Source: CAD feature listing. Evaluate the final solid. Frame: model axes, mm. Face numbers are marked on the shaded views. A direction names the side the tool comes from. Round coordinates to 2 decimals unless told otherwise and drop trailing zeros. Write each loop counter-clockwise with the first axis right and the second up, starting at its lowest first coordinate (ties: lowest second). Pieces come first, ordered by that corner, then holes. Notation, with made-up numbers: (81, -21) -> (89, -21) arc R32 ccw to (89, 9) -> close; hole circle Ø8 at (25.5, 44). An arc over 180 degrees is marked (long way). Put each result on its own line as item: value.
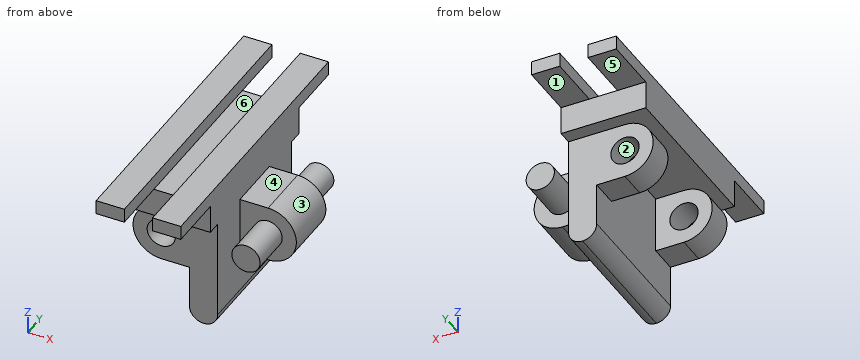
```python
from build123d import *

# Parameters (mm, degrees)
F0_W      = 5
F0_H      = 10
F0_R      = 2.5
F1_DEPTH  = 12.5
F2_DEPTH  = 5
F3_DEPTH  = 12.5
F4_DEPTH  = 7.5
F7_DEPTH  = 10
F8_R      = 2.5
F9_R      = 2.49999
F10_W     = 15
F10_H     = 30
F11_DEPTH = 5
F12_W     = 5
F12_H     = 50
F13_DEPTH = 2.5


# Not quite as in the source:
# - a fillet or chamfer is up to 0.001 mm smaller than in the source, because OpenCascade refuses the exact size


with BuildPart() as f1:
    # F0 (on Front) → F1 (new body)
    with BuildSketch(Plane.XZ):
        with Locations((7.5, 0)):
            Rectangle(F0_W, F0_H)
        with BuildLine():
            Line((5, 5), (0, 5))
            ThreePointArc((0, 5), (-5, 0), (0, -5))
            Line((0, -5), (5, -5))
            Line((5, -5), (5, 5))
        make_face()
        Circle(F0_R, mode=Mode.SUBTRACT)
    extrude(amount=F1_DEPTH)

    # F0 (on Front) → F2 (join)
    with BuildSketch(Plane.XZ):
        with BuildLine():
            Line((15, 5), (10, 5))
            Line((10, 5), (10, -5))
            Line((10, -5), (15, -5))
            ThreePointArc((15, -5), (20, 0), (15, 5))
        make_face()
        with Locations((15, 0)):
            Circle(F0_R, mode=Mode.SUBTRACT)
    extrude(amount=F2_DEPTH)

    # F0 (on Front) → F3 (join)
    with BuildSketch(Plane.XZ):
        with Locations((15, 0)):
            Circle(F0_R)
    extrude(amount=F3_DEPTH)

    # F0 (on Front) → F4 (cut)
    with BuildSketch(Plane.XZ):
        with BuildLine():
            Line((5, 5), (0, 5))
            ThreePointArc((0, 5), (-5, 0), (0, -5))
            Line((0, -5), (5, -5))
            Line((5, -5), (5, 5))
        make_face()
        Circle(F0_R, mode=Mode.SUBTRACT)
    extrude(amount=F4_DEPTH, mode=Mode.SUBTRACT)

    # F5: F1 across plane


with BuildPart() as f1_1:
    add(f1.part)
    add(f1.part.mirror(Plane.XZ))

    # F6 (on face) → F7 (join)
    with BuildSketch(Plane(origin=(0, 0, -5), x_dir=(1, 0, 0), z_dir=(0, 0, -1))):
        Polygon((10, 5), (10, 12.5), (5, 12.5), (5, 7.5), (5, -7.5), (5, -12.5), (10, -12.5), (10, -5), align=None)
    extrude(amount=F7_DEPTH)

    # F8
    f8_edges = [f1_1.edges().sort_by_distance(p)[0] for p in [
        (10, 0, -15),
    ]]
    fillet(f8_edges, radius=F8_R)

    # F9 (radius 2.5 in the source; OpenCascade refuses exactly that, so slightly less here)
    f9_edges = [f1_1.edges().sort_by_distance(p)[0] for p in [
        (5, 0, -15),
    ]]
    fillet(f9_edges, radius=F9_R)

    # F10 (on face) → F11 (join)
    with BuildSketch(Plane.XY.offset(5)):
        with Locations((2.5, 0)):
            Rectangle(F10_W, F10_H)
    extrude(amount=F11_DEPTH)

    # F12 (on face) → F13 (join)
    with BuildSketch(Plane.XY.offset(10)):
        with Locations((-2.5, 0)):
            Rectangle(F12_W, F12_H)
        with Locations((7.5, 0)):
            Rectangle(F12_W, F12_H)
    extrude(amount=F13_DEPTH)


solid = f1_1.part
```
Q1. Cut plane A-A on z = 0. Output: boundary loops of the cut face in (x, y), and give its area (3 significant figures).
Ans:
outline: (-5, -12.5) -> (-2.5, -12.5) -> (-2.5, -7.5) -> (-5, -7.5) -> close; (-5, 7.5) -> (-2.5, 7.5) -> (-2.5, 12.5) -> (-5, 12.5) -> close; (2.5, -12.5) -> (10, -12.5) -> (10, -5) -> (12.5, -5) -> (12.5, -12.5) -> (17.5, -12.5) -> (17.5, -5) -> (20, -5) -> (20, 5) -> (17.5, 5) -> (17.5, 12.5) -> (12.5, 12.5) -> (12.5, 5) -> (10, 5) -> (10, 12.5) -> (2.5, 12.5) -> (2.5, 7.5) -> (5, 7.5) -> (5, -7.5) -> (2.5, -7.5) -> close
area: 350 mm^2
Q2. Cut plane B-B on y = 19. Output: boundary loops of the cut face in (x, z).
Ans:
outline: (-5, 10) -> (0, 10) -> (0, 12.5) -> (-5, 12.5) -> close; (5, 10) -> (10, 10) -> (10, 12.5) -> (5, 12.5) -> close
Q3. Material intervals for line 1 (X direction, y = -10, z = 11.25); line 2 (Z direction, x = 4.75, y = -13); line 3 (Y direction, x = -3.5, z = 3.25), sorted ascending. Write a range as [from, to].
Ans:
line 1: x = [-5, 0], [5, 10]
line 2: z = [5, 10]
line 3: y = [-12.5, -7.5], [7.5, 12.5]
Q4. Reachability of the marked faces 4, 5 and 6 from +Z, -Z, +X, -X, +Y, -Y: full face, straight path, thin tool, end or side. Return the list, or none.
Ans:
face 4: +Z, +X, +Y, -Y
face 5: -Z, +X, -X, +Y
face 6: +Z, +Y, -Y
Q5. Pin query (flat end, axial travel): pin 1 (11 mm diameter, centred on x = 1, z = -1.5, fed in from -Y); pin 2 (12 mm diameter, centred on x = 4, z = 9.5, fed in from -Y); pin 3 (4 mm diameter, centred on x = -3.5, y = 20.5, fed in from -Z); pin 4 (3 mm diameter, centred on x = 4, y = 15, fed in from -Z). Return the tip coordinate at first contact, or that it passes through.
Ans:
pin 1: stops at y = -12.5
pin 2: stops at y = -25
pin 3: stops at z = 10
pin 4: stops at z = 5
Q6. Draft query along X for the marked faces 1, 2 and 3. Return one class per face: +X half, -X half, draft (parallel to the pull), parting line (faces both ways), or undercut.
Ans:
face 1: draft
face 2: undercut
face 3: +X half
Q7. Cut plane C-C on x = -1. Output: boundary loops of the cut face in (y, z), and give its area (3 significant figures).
Ans:
outline: (-25, 10) -> (-15, 10) -> (-15, 5) -> (15, 5) -> (15, 10) -> (25, 10) -> (25, 12.5) -> (-25, 12.5) -> close; (-12.5, -4.9) -> (-7.5, -4.9) -> (-7.5, -2.29) -> (-12.5, -2.29) -> close; (-12.5, 2.29) -> (-7.5, 2.29) -> (-7.5, 4.9) -> (-12.5, 4.9) -> close; (7.5, -4.9) -> (12.5, -4.9) -> (12.5, -2.29) -> (7.5, -2.29) -> close; (7.5, 2.29) -> (12.5, 2.29) -> (12.5, 4.9) -> (7.5, 4.9) -> close
area: 327 mm^2
